```python
from build123d import *

# Parameters (mm, degrees)
SKETCH1_R           = 3.571875
BOSS_EXTRUDE1_DEPTH = 0.9525
SKETCH2_R           = 1.4605
BOSS_EXTRUDE2_DEPTH = 6.35


with BuildPart() as part:
    # Sketch1 → Boss-Extrude1 (new body)
    with BuildSketch(Plane(origin=(0, 0, 0), x_dir=(1, 0, 0), z_dir=(0, 1, 0))):
        with Locations(Location((0, 0, 0), (0, 0, 90))):
            Circle(SKETCH1_R)
    extrude(amount=BOSS_EXTRUDE1_DEPTH)

    # Sketch2 → Boss-Extrude2 (add)
    with BuildSketch(Plane(origin=(0, 0.9525, 0), x_dir=(1, 0, 0), z_dir=(0, 1, 0))):
        with Locations(Location((0, 0, 0), (0, 0, 270))):
            Circle(SKETCH2_R)
    extrude(amount=BOSS_EXTRUDE2_DEPTH)

    # Sketch3 → Cut-Revolve1 (revolve, cut)
    with BuildSketch(Plane(origin=(0, 0, 0), x_dir=(0, 0, -1), z_dir=(1, 0, 0))):
        Polygon((-1.4605, 0.9525), (-1.2065, 7.3025), (-1.4605, 7.3025), (-1.738282531, 7.3025), align=None)
    revolve(axis=Axis((0, 7.3025, 0), (0, -1, 0)), mode=Mode.SUBTRACT)


solid = part.part
```
Here's how the part is built. I have some questions about the finished solid (model axes, mm). A direction names the side the tool comes from. Coordinates: 2 decimals unless noted, no trailing zeros. Order: outer loops, then holes, each group sorted by start corner. A loop starts at its lowest first (then second) coordinate and runs counter-clockwise, first axis right, second up.
1) Will these pins go through, and if not, where does the flat tip stop? pin 1 (2 mm diameter, centred on x = -1.5, z = 0, fed in from -Y); pin 2 (3 mm diameter, centred on x = 1.5, y = 3.5, fed in from +Z); pin 3 (1.5 mm diameter, centred on x = 0.5, y = 6.5, fed in from +Z); pin 4 (1 mm diameter, centred on x = 1.5, z = -2.5, fed in from +Y).
2) Which directions (+Z, -Z, +X, -X, +Y, -Y) give clear straight access to the entire face, cutting with the end or side of a thin tool? Please do faces 1 (the face through (0, 0, 0)), 2 (the face through (2, 0.952, 0)).
3) Imagine slicing it at C-C on y = 2.5. List the corners of the cut face in (x, z) for me.
4) Imagine slicing it at B-B on x = 0. List the corners of the cut face in (y, z) for me, and give its area (3 significant figures).
5) I need wall thicknesses on line 1 (Y direction, x = 2.5, z = -2.25); line 2 (X direction, y = 3.75, z = 0); line 3 (Z direction, x = -0.75, y = 3.5). Which ranges of each line are inside material? Lowest first, please.
6) Imagine slicing it at A-A on z = 0. List the corners of the cut face in (x, y) for me, and give its area (3 significant figures).
7) Imagine slicing it at D-D on z = 3.25. List the corners of the cut face in (x, y) for me, and give its area (3 significant figures).
Response values:
1. pin 1: stops at y = 0
1. pin 2: stops at z = 1.38
1. pin 3: stops at z = 1.26
1. pin 4: stops at y = 0.95
2. face 1: +Z, -Z, +X, -X, -Y
2. face 2: +Y
3. outline: circle Ø2.8 at (0, 0)
4. outline: (0, -3.57) - (0.95, -3.57) - (0.95, -1.46) - (7.3, -1.21) - (7.3, 1.21) - (0.95, 1.46) - (0.95, 3.57) - (0, 3.57) - close
4. area: 23.7 mm2
5. line 1: y = 0 to 0.95
5. line 2: x = -1.35 to 1.35
5. line 3: z = -1.13 to 1.13
6. outline: (-3.57, 0) - (3.57, 0) - (3.57, 0.95) - (1.46, 0.95) - (1.21, 7.3) - (-1.21, 7.3) - (-1.46, 0.95) - (-3.57, 0.95) - close
6. area: 23.7 mm2
7. outline: (-1.48, 0) - (1.48, 0) - (1.48, 0.95) - (-1.48, 0.95) - close
7. area: 2.82 mm2
